Input: part model. Units: mm. Frame: model coordinates. Coordinates: 2 decimals unless noted, no trailing zeros. Loops run counter-clockwise (first coordinate to the right, second up) from the corner with the lowest first, then second, coordinate; pieces in that order, holes last. Notation, with made-up numbers: (66.5, -35.75) - (74.5, -35.75) arc R15 cw to (74.5, -16.75) - close; hole circle Ø11 at (-28, 2). An arc over 180 degrees is marked (long way). Use one line per item in the form item = value.
from build123d import *

# Parameters (mm, degrees)
CROQUIS12_W           = 115
CROQUIS12_H           = 329.4
BRIDA_BASE2_DEPTH     = 1.5
CORTAR_EXTRUIR6_REACH = 217.797
CROQUIS27_R           = 2
CORTAR_EXTRUIR7_REACH = 217.797
CROQUIS28_R           = 7.5
CROQUIS29_W           = 16
CROQUIS29_H           = 35
CORTAR_EXTRUIR8_DEPTH = 216.796988162
REDONDEO1_R           = 6
REDONDEO2_R           = 2


# Sheet-metal steps are written as plain solids
with BuildPart() as part:
    # Croquis12 → Brida base2 (new body)
    with BuildSketch(Plane(origin=(0, 0, 0), x_dir=(1, 0, 0), z_dir=(0, 1, 0))):
        with Locations((0, -43.29)):
            Rectangle(CROQUIS12_W, CROQUIS12_H)
    extrude(amount=-BRIDA_BASE2_DEPTH)

    # Croquis27 → Cortar-Extruir6 (cut, up to next)
    with BuildSketch(Plane(origin=(0, 0, 0), x_dir=(1, 0, 0), z_dir=(0, 1, 0)), mode=Mode.PRIVATE) as cortar_extruir6_sk1:
        with Locations(Location((-53.5, -201.3, 0), (0, 0, 270))):
            Circle(CROQUIS27_R)
    cortar_extruir6_tool1 = extrude(cortar_extruir6_sk1.sketch, amount=-CORTAR_EXTRUIR6_REACH, mode=Mode.PRIVATE) & part.part
    # Croquis27 → Cortar-Extruir6 (cut, up to next)
    with BuildSketch(Plane(origin=(0, 0, 0), x_dir=(1, 0, 0), z_dir=(0, 1, 0)), mode=Mode.PRIVATE) as cortar_extruir6_sk2:
        with Locations(Location((-53.5, 78.26, 0), (0, 0, 270))):
            Circle(CROQUIS27_R)
    cortar_extruir6_tool2 = extrude(cortar_extruir6_sk2.sketch, amount=-CORTAR_EXTRUIR6_REACH, mode=Mode.PRIVATE) & part.part
    # Croquis27 → Cortar-Extruir6 (cut, up to next)
    with BuildSketch(Plane(origin=(0, 0, 0), x_dir=(1, 0, 0), z_dir=(0, 1, 0)), mode=Mode.PRIVATE) as cortar_extruir6_sk3:
        with Locations(Location((53.5, 78.26, 0), (0, 0, 90))):
            Circle(CROQUIS27_R)
    cortar_extruir6_tool3 = extrude(cortar_extruir6_sk3.sketch, amount=-CORTAR_EXTRUIR6_REACH, mode=Mode.PRIVATE) & part.part
    # Croquis27 → Cortar-Extruir6 (cut, up to next)
    with BuildSketch(Plane(origin=(0, 0, 0), x_dir=(1, 0, 0), z_dir=(0, 1, 0)), mode=Mode.PRIVATE) as cortar_extruir6_sk4:
        with Locations(Location((53.5, -201.3, 0), (0, 0, 90))):
            Circle(CROQUIS27_R)
    cortar_extruir6_tool4 = extrude(cortar_extruir6_sk4.sketch, amount=-CORTAR_EXTRUIR6_REACH, mode=Mode.PRIVATE) & part.part
    add(cortar_extruir6_tool1.solids().sort_by_distance((-53.5, 0, 201.3))[0], mode=Mode.SUBTRACT)
    add(cortar_extruir6_tool2.solids().sort_by_distance((-53.5, 0, -78.26))[0], mode=Mode.SUBTRACT)
    add(cortar_extruir6_tool3.solids().sort_by_distance((53.5, 0, -78.26))[0], mode=Mode.SUBTRACT)
    add(cortar_extruir6_tool4.solids().sort_by_distance((53.5, 0, 201.3))[0], mode=Mode.SUBTRACT)

    # Croquis28 → Cortar-Extruir7 (cut, up to next)
    with BuildSketch(Plane(origin=(0, 0, 0), x_dir=(1, 0, 0), z_dir=(0, 1, 0)), mode=Mode.PRIVATE) as cortar_extruir7_sk1:
        with Locations(Location((0, 96.25, 0), (0, 0, 270))):
            Circle(CROQUIS28_R)
    cortar_extruir7_tool1 = extrude(cortar_extruir7_sk1.sketch, amount=-CORTAR_EXTRUIR7_REACH, mode=Mode.PRIVATE) & part.part
    add(cortar_extruir7_tool1.solids().sort_by_distance((0, 0, -96.25))[0], mode=Mode.SUBTRACT)

    # Croquis29 → Cortar-Extruir8 (cut, through all)
    with BuildSketch(Plane(origin=(0, 0, 0), x_dir=(1, 0, 0), z_dir=(0, 1, 0))):
        with Locations((39, 103.91)):
            Rectangle(CROQUIS29_W, CROQUIS29_H)
    extrude(amount=-CORTAR_EXTRUIR8_DEPTH, mode=Mode.SUBTRACT)

    # Redondeo1
    redondeo1_edges = [part.edges().sort_by_distance(p)[0] for p in [
        (31, -0.75, -86.41),
        (47, -0.75, -86.41),
    ]]
    fillet(redondeo1_edges, radius=REDONDEO1_R)

    # Redondeo2
    redondeo2_edges = [part.edges().sort_by_distance(p)[0] for p in [
        (31, -0.75, -121.41),
        (47, -0.75, -121.41),
    ]]
    fillet(redondeo2_edges, radius=REDONDEO2_R)


solid = part.part
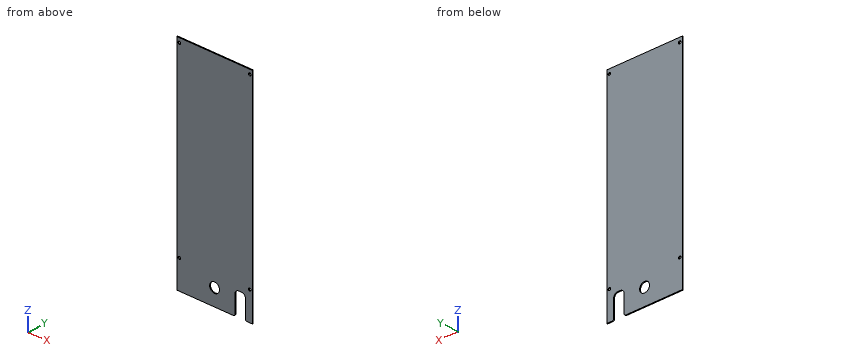
Q1. Cut plane A-A, the plane z = -96.25. Return loops of the section in (x, y).
Check values:
outline = (-57.5, -1.5) - (-7.5, -1.5) - (-7.5, 0) - (-57.5, 0) - close; (7.5, -1.5) - (31, -1.5) - (31, 0) - (7.5, 0) - close; (47, -1.5) - (57.5, -1.5) - (57.5, 0) - (47, 0) - close
Q2. Cut plane C-C, the plane y = -1.05. Return loops of the section in (x, z).
Check values:
outline = (-57.5, -121.41) - (29, -121.41) arc R2 ccw to (31, -119.41) - (31, -92.41) arc R6 cw to (37, -86.41) - (41, -86.41) arc R6 cw to (47, -92.41) - (47, -119.41) arc R2 ccw to (49, -121.41) - (57.5, -121.41) - (57.5, 207.99) - (-57.5, 207.99) - close; hole circle Ø4 at (-53.5, -78.26); hole circle Ø4 at (-53.5, 201.3); hole circle Ø15 at (0, -96.25); hole circle Ø4 at (53.5, -78.26); hole circle Ø4 at (53.5, 201.3)
Q3. Cut plane B-B, the plane x = 0. Return loops of the section in (y, z), then the cut area to 3 significant figures.
Check values:
outline = (-1.5, -121.41) - (0, -121.41) - (0, -103.75) - (-1.5, -103.75) - close; (-1.5, -88.75) - (0, -88.75) - (0, 207.99) - (-1.5, 207.99) - close
area = 472 mm²
Q4. Ray query, line 1 along X through (y, z) = (-0.5, -78.26); line 2 along Z through (x, y) = (53.5, -0.6); line 3 along Z through (x, y) = (6.5, -0.7). Return the intervals inside material, ascending. Write a range as [from, to].
Check values:
line_1 = [-57.5, -55.5], [-51.5, 51.5], [55.5, 57.5]
line_2 = [-121.41, -80.26], [-76.26, 199.3], [203.3, 207.99]
line_3 = [-121.41, -99.99], [-92.51, 207.99]
